Could you check a few things on this model? Use its own coordinates, in mm. Face numbers are marked on the shaded views. A direction names the side the tool comes from. Give positions to 0.01 mm unless a question says otherwise; leave off trailing zeros. Order: outer loops, then holes, each group sorted by start corner. A loop starts at its lowest first (then second) coordinate and runs counter-clockwise, first axis right, second up.
(1) Will these pins go through, and if not, where does the flat tip stop? pin 1 (1.5 mm diameter, centred on x = 21.5, z = 6.5, fed in from +Y); pin 2 (1.8 mm diameter, centred on x = 6.5, z = 3.5, fed in from +Y); pin 3 (1.5 mm diameter, centred on x = 14, y = 5.5, fed in from +Z).
(2) On a 3-axis mill with a long thin cutter (end or side, diameter ignored), from which of +Z, -Z, +X, -X, +Y, -Y can I reach the whole of each face in a straight line? I mean the marked faces 1, 2 and 3. Say none if no direction works.
(3) Imagine slicing it at D-D, the plane x = 29. Write out the boundary of the cut face in (y, z).
(4) Imagine slicing it at C-C, the plane x = 37.5. Write out the boundary of the cut face in (y, z), then the cut area to 3 significant figures.
(5) Imagine slicing it at A-A, the plane z = 2.75. Write out the boundary of the cut face in (x, y).
(6) If I drill on probe 1 along X at (y, z) = (0.25, 7); probe 2 along Y at (x, z) = (22, 4.5); probe 3 along Y at (x, z) = (21, 5), over which ranges is the centre line in solid material (lowest first)?
(7) Imagine slicing it at B-B, the plane y = 0. Write out the boundary of the cut face in (x, z).
from build123d import *

# Parameters (mm, degrees)
SKETCH1_R           = 1.5
BOSS_EXTRUDE1_DEPTH = 8
FILLET1_R           = 1


with BuildPart() as part:
    # Sketch1 → Boss-Extrude1 (new body)
    with BuildSketch(Plane.XY):
        with BuildLine():
            Line((20.05, 5), (0, 5))
            ThreePointArc((0, 5), (-5, 0), (0, -5))
            Line((0, -5), (22, -5))
            Line((22, -5), (26.640289064, 1.862180818))
            ThreePointArc((26.640289064, 1.862180818), (24.800812017, 4.141914056), (22, 5))
            Line((22, 5), (20.05, 5))
        make_face()
        Circle(SKETCH1_R, mode=Mode.SUBTRACT)
        with Locations((22, 0)):
            Circle(SKETCH1_R, mode=Mode.SUBTRACT)
        with BuildLine():
            Line((46.409029503, 15.837507263), (20.05, 5))
            Line((20.05, 5), (22, 5))
            ThreePointArc((22, 5), (24.800812017, 4.141914056), (26.640289064, 1.862180818))
            Line((26.640289064, 1.862180818), (36.049561342, 5.638188326))
            Line((36.049561342, 5.638188326), (42.488975113, 3.018953392))
            Line((42.488975113, 3.018953392), (43.653419291, 2.816543521))
            Line((43.653419291, 2.816543521), (44.338731569, 3.779480217))
            Line((44.338731569, 3.779480217), (45.503175747, 3.577070346))
            Line((45.503175747, 3.577070346), (46.188488025, 4.540007042))
            Line((46.188488025, 4.540007042), (47.352932204, 4.337597171))
            Line((47.352932204, 4.337597171), (48.038244482, 5.300533868))
            Line((48.038244482, 5.300533868), (49.20268866, 5.098123997))
            Line((49.20268866, 5.098123997), (49.888000938, 6.061060693))
            Line((49.888000938, 6.061060693), (51.052445116, 5.858650822))
            Line((51.052445116, 5.858650822), (51.737757394, 6.821587519))
            Line((51.737757394, 6.821587519), (52.902201573, 6.619177648))
            Line((52.902201573, 6.619177648), (53.587513851, 7.582114344))
            Line((53.587513851, 7.582114344), (54.751958029, 7.379704473))
            Line((54.751958029, 7.379704473), (55.437270307, 8.34264117))
            Line((55.437270307, 8.34264117), (53.72608495, 12.504593197))
            Line((53.72608495, 12.504593197), (46.409029503, 15.837507263))
        make_face()
    extrude(amount=BOSS_EXTRUDE1_DEPTH)

    # Fillet1
    fillet1_edges = [part.edges().sort_by_distance(p)[0] for p in [
        (11, -5, 8),
        (11, -5, 0),
        (-5, 0, 0),
        (10.025, 5, 0),
        (10.025, 5, 8),
        (-5, 0, 8),
    ]]
    fillet(fillet1_edges, radius=FILLET1_R)


solid = part.part
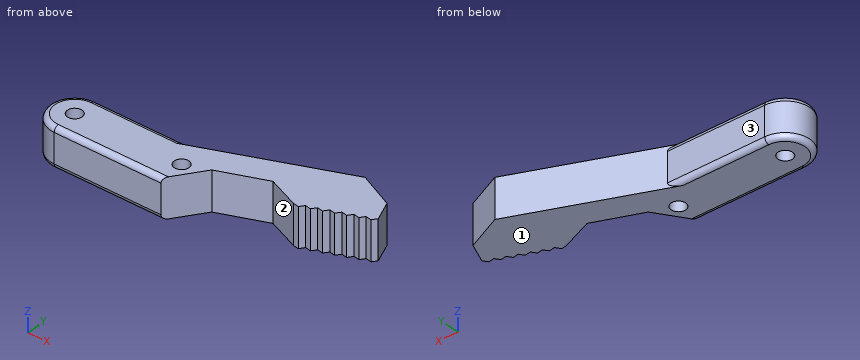
Answer block:
1. pin 1: stops at y = 5.9
1. pin 2: stops at y = 5
1. pin 3: stops at z = 7.66
2. face 1: -Z, +X, -X, +Y, -Y
2. face 2: +Z, -Z, -Y
2. face 3: +Z, -Z, -X, +Y
3. outline: (2.81, 0) - (8.68, 0) - (8.68, 8) - (2.81, 8) - close
4. outline: (5.05, 0) - (12.17, 0) - (12.17, 8) - (5.05, 8) - close
4. area: 57.0 mm2
5. outline: (0, -5) - (22, -5) - (26.64, 1.86) - (36.05, 5.64) - (42.49, 3.02) - (43.65, 2.82) - (44.34, 3.78) - (45.5, 3.58) - (46.19, 4.54) - (47.35, 4.34) - (48.04, 5.3) - (49.2, 5.1) - (49.89, 6.06) - (51.05, 5.86) - (51.74, 6.82) - (52.9, 6.62) - (53.59, 7.58) - (54.75, 7.38) - (55.44, 8.34) - (53.73, 12.5) - (46.41, 15.84) - (20.05, 5) - (0, 5) arc R5 ccw to start; hole circle Ø3 at (0, 0); hole circle Ø3 at (22, 0)
6. probe 1: x = -4.99 to -1.48, 1.48 to 20.52, 23.48 to 25.55
6. probe 2: y = -5 to -1.5, 1.5 to 5.8
6. probe 3: y = -5 to -1.12, 1.12 to 5.39
7. outline: (-5, 1) arc R1 ccw to (-4, 0) - (-1.5, 0) - (-1.5, 8) - (-4, 8) arc R1 ccw to (-5, 7) - close; (1.5, 0) - (20.5, 0) - (20.5, 8) - (1.5, 8) - close; (23.5, 0) - (25.38, 0) - (25.38, 8) - (23.5, 8) - close
